from build123d import *

# Parameters (mm, degrees)
SKETCH1_R              = 4.7625
BOSS_EXTRUDE1_DEPTH    = 438.15
SKETCH2_W              = 7.873653068
SKETCH2_H              = 76.2
BOSS_EXTRUDE2_DEPTH    = 11.90625
FILLET1_R              = 12.7
LPATTERN1_COUNT        = 2
LPATTERN1_PITCH        = 82.55
LPATTERN1_COUNT_DIR2   = 2
LPATTERN1_PITCH_DIR2   = 82.55
FILLET1_OF_LPATTERN1_R = 12.7


with BuildPart() as part:
    # Sketch1 → Boss-Extrude1 (new body)
    with BuildSketch(Plane.XY):
        Circle(SKETCH1_R)
    extrude(amount=BOSS_EXTRUDE1_DEPTH)

    # Sketch2 → Boss-Extrude2 (add, symmetric)
    with BuildSketch(Plane.XY.offset(219.075)):
        with Locations((0, -6.35)):
            Rectangle(SKETCH2_W, SKETCH2_H)
    boss_extrude2 = extrude(amount=BOSS_EXTRUDE2_DEPTH, both=True)

    # Fillet1
    # the kernel refuses this fillet: 12.7 mm, written as the material it takes off along each edge
    with BuildSketch(Plane(origin=(35.686826534, 31.75, 207.16875), x_dir=(0, -1, 0), z_dir=(-1, 0, 0)), Plane(origin=(-35.686826534, -44.45, 207.16875), x_dir=(0, 1, 0), z_dir=(1, 0, 0))) as fillet1_piece_1:
        with BuildLine():
            CenterArc((FILLET1_R, FILLET1_R), FILLET1_R, 180, 90)
            Line((0, FILLET1_R), (0, 0))
            Line((0, 0), (FILLET1_R, 0))
        make_face()
    extrude(amount=71.373653068, mode=Mode.SUBTRACT)
    with BuildSketch(Plane(origin=(35.686826534, 31.75, 230.98125), x_dir=(0, -1, 0), z_dir=(-1, 0, 0)), Plane(origin=(-35.686826534, -44.45, 230.98125), x_dir=(0, 1, 0), z_dir=(1, 0, 0))) as fillet1_piece_2:
        with BuildLine():
            CenterArc((FILLET1_R, -FILLET1_R), FILLET1_R, 90, 90)
            Line((0, -FILLET1_R), (0, 0))
            Line((0, 0), (FILLET1_R, 0))
        make_face()
    extrude(amount=71.373653068, mode=Mode.SUBTRACT)

    # LPattern1: Boss-Extrude2 2 × 2
    with Locations(*[Vector(0, 0, 1) * (i * LPATTERN1_PITCH) + Vector(0, 0, -1) * (j * LPATTERN1_PITCH_DIR2) for i in range(LPATTERN1_COUNT) for j in range(LPATTERN1_COUNT_DIR2) if (i, j) != (0, 0)]):
        add(boss_extrude2)

    # Fillet1 of LPattern1
    # the kernel refuses this fillet: 12.7 mm, written as the material it takes off along each edge
    with BuildSketch(Plane(origin=(35.686826534, 31.75, 124.61875), x_dir=(0, 0, 1), z_dir=(-1, 0, 0)), Plane(origin=(35.686826534, 31.75, 289.71875), x_dir=(0, 0, 1), z_dir=(-1, 0, 0)), Plane(origin=(35.686826534, 31.75, 313.53125), x_dir=(0, -1, 0), z_dir=(-1, 0, 0)), Plane(origin=(-35.686826534, -44.45, 289.71875), x_dir=(0, 0, 1), z_dir=(1, 0, 0)), Plane(origin=(35.686826534, 31.75, 207.16875), x_dir=(0, 0, 1), z_dir=(-1, 0, 0))) as fillet1_of_lpattern1_piece_1:
        with BuildLine():
            CenterArc((FILLET1_OF_LPATTERN1_R, -FILLET1_OF_LPATTERN1_R), FILLET1_OF_LPATTERN1_R, 90, 90)
            Line((0, -FILLET1_OF_LPATTERN1_R), (0, 0))
            Line((0, 0), (FILLET1_OF_LPATTERN1_R, 0))
        make_face()
    extrude(amount=71.373653068, mode=Mode.SUBTRACT)
    with BuildSketch(Plane(origin=(35.686826534, 31.75, 148.43125), x_dir=(0, 0, -1), z_dir=(-1, 0, 0)), Plane(origin=(-35.686826534, -44.45, 148.43125), x_dir=(0, 0, -1), z_dir=(1, 0, 0)), Plane(origin=(-35.686826534, -44.45, 124.61875), x_dir=(0, 1, 0), z_dir=(1, 0, 0)), Plane(origin=(-35.686826534, -44.45, 313.53125), x_dir=(0, 0, -1), z_dir=(1, 0, 0)), Plane(origin=(35.686826534, 31.75, 230.98125), x_dir=(0, 0, -1), z_dir=(-1, 0, 0)), Plane(origin=(-35.686826534, -44.45, 230.98125), x_dir=(0, 0, -1), z_dir=(1, 0, 0)), Plane(origin=(-35.686826534, -44.45, 207.16875), x_dir=(0, 1, 0), z_dir=(1, 0, 0))) as fillet1_of_lpattern1_piece_2:
        with BuildLine():
            CenterArc((FILLET1_OF_LPATTERN1_R, FILLET1_OF_LPATTERN1_R), FILLET1_OF_LPATTERN1_R, 180, 90)
            Line((0, FILLET1_OF_LPATTERN1_R), (0, 0))
            Line((0, 0), (FILLET1_OF_LPATTERN1_R, 0))
        make_face()
    extrude(amount=71.373653068, mode=Mode.SUBTRACT)


solid = part.part
CAD build for the part. Positions are in the model's coordinates, mm. A direction names the side the tool comes from. Coordinates: 2 decimals unless noted, no trailing zeros. Loops run counter-clockwise (first coordinate to the right, second up) from the corner with the lowest first, then second, coordinate; pieces in that order, holes last. Notation, with made-up numbers: (12.25, -6.75) - (28.25, -6.75) arc R29 cw to (28.25, 30.25) - close; hole circle Ø11 at (53.25, 65.5). An arc over 180 degrees is marked (long way). Write item = value, one per line. Start each with the question number.
Q1. Cut at C-C, the plane z = 341. List the corners of the cut face in (x, y) (1 decimal), then the cut area to 3 significant figures.
Q2. Cut at A-A, the plane y = -18. List the corners of the cut face in (x, z).
Q3. Which spindle directions (+Z, -Z, +X, -X, +Y, -Y) get a long thin tool onto all of the face, cutting with end or side? Do faces 1 (the cylindrical face through (4.543, 1.431, 216.008)), 2 (the cylindrical face through (-0.06, -40.54, 210.7)), 3 (the cylindrical face through (0.06, 27.84, 293.25)), 4 (the flat face through (-3.937, 17, 302)). Say none if no direction does.
Q4. Drill centre lines: L1, parallel to Z at x = 1, y = -29.5; L2, parallel to X at y = -28, z = 212.5; L3, parallel to Y at x = 0.75, z = 257. Where is each one in solid material? Low to high.
Q5. Flat gauge pins, fed straight in: pin 1 Ø12 at (y, z) = (-19, 298) entering from -X; pin 2 Ø4 at (x, y) = (1.5, -17.5) entering from -Z; pin 3 Ø12 at (y, z) = (14.5, 136.5) entering from +X; pin 4 Ø2 at (x, y) = (3.5, 3) entering from -Z. Where does each tip first touch, or does it go through?
Q6. Cut at D-D, the plane y = 24. List the corners of the cut face in (x, z), then the cut area to 3 significant figures.
Computed:
q1.outline = circle Ø9.5 at (0, 0)
q1.area = 71.3 mm²
q2.outline = (-3.94, 124.62) - (3.94, 124.62) - (3.94, 148.43) - (-3.94, 148.43) - close; (-3.94, 207.17) - (3.94, 207.17) - (3.94, 230.98) - (-3.94, 230.98) - close; (-3.94, 289.72) - (3.94, 289.72) - (3.94, 313.53) - (-3.94, 313.53) - close
q3.face_1 = none
q3.face_2 = +X, -X, -Y
q3.face_3 = +X, -X, +Y
q3.face_4 = +Z, -Z, -X, +Y
q4.L1 = 124.62 to 148.43, 207.17 to 230.98, 289.72 to 313.53
q4.L2 = -3.94 to 3.94
q4.L3 = -4.7 to 4.7
q5.pin_1 = -3.94
q5.pin_2 = 124.62
q5.pin_3 = 3.94
q5.pin_4 = 0
q6.outline = (-3.94, 125.62) - (3.94, 125.62) - (3.94, 147.43) - (-3.94, 147.43) - close; (-3.94, 208.17) - (3.94, 208.17) - (3.94, 229.98) - (-3.94, 229.98) - close; (-3.94, 290.72) - (3.94, 290.72) - (3.94, 312.53) - (-3.94, 312.53) - close
q6.area = 515 mm²
